Work out the finished part from the listing and answer in its coordinate system (mm). A direction names the side the tool comes from. Round coordinates to 2 decimals unless told otherwise and drop trailing zeros. Loops run counter-clockwise (first coordinate to the right, second up) from the corner with the lowest first, then second, coordinate; pieces in that order, holes last.
Autodesk Inventor part; units mm, degrees
ref_plane "YZ Plane" through (0, 0, 0) normal (1, 0, 0) x (0, 1, 0)
ref_plane "XZ Plane" through (0, 0, 0) normal (0, 1, 0) x (-1, 0, 0)
sketch "Sketch1" plane through (0, 0, 0) normal (0, 1, 0) x (-1, 0, 0)
  line L0 (-20, 10) -> (20, 10)
  line L1 (20, 10) -> (20, -10)
  line L2 (20, -10) -> (-20, -10)
  line L3 (-20, -10) -> (-20, 10)
  line L4 (-20, 10) -> (20, -10) construction
  line L5 (20, 10) -> (-20, -10) construction
  point P0 (0, 0)
  dimension "d0" = 40
  dimension "d1" = 20
extrude "Extrusion1" add sketch "Sketch1" along normal blind 37
sketch "Sketch2" plane through (0, 37, 0) normal (0, 1, 0) x (1, 0, 0)
  line L0 (20, 10) -> (-20, 10)
  line L1 (-20, 10) -> (-20, -10)
  line L2 (-20, -10) -> (20, -10)
  line L3 (20, -10) -> (20, 10)
  circle A0 centre (-10, 0) radius 10
  line L4 (-20, 10) -> (-20, -10)
  line L5 (15, -10) -> (15, 10)
  line L6 (15, 9.25) -> (-6.2003, 9.25)
  line L7 (-6.2003, -9.25) -> (15, -9.25)
  point P0 (0, 0)
  dimension "d4" = 5
extrude "Extrusion2" add sketch "Sketch2" along normal blind 2 contours A0 | L5 L7 A0 L6
sketch "Sketch3" plane through (0, 39, 0) normal (0, 1, 0) x (1, 0, 0)
  line L0 (-6.2003, -9.25) -> (15, -9.25)
  line L1 (15, -9.25) -> (15, 9.25)
  line L2 (15, 9.25) -> (-6.2003, 9.25)
  arc A0 (-6.2003, 9.25) -> (-6.2003, -9.25) centre (-10, 0) ccw
  circle A1 centre (-10, 0) radius 6.5
  point P0 (0, 0)
  dimension "d8" = 13
extrude "Extrusion3" add sketch "Sketch3" along normal blind 2 contours A1
sketch "Sketch4" plane through (-10, 41, 0) normal (0, 1, 0) x (1, 0, 0)
  circle A0 centre (0, 0) radius 6.5
  circle A1 centre (0, 0) radius 2.9
  circle A2 centre (0, 0) radius 1.5
  point P0 (10, 0)
  dimension "d11" = 5.8
  dimension "d12" = 3
extrude "Extrusion4" add sketch "Sketch4" along normal blind 4 contours A1
ref_plane "Work Plane1" through (0, 28, 0) normal (0, -1, 0) x (1, 0, 0)
sketch "Sketch5" plane through (0, 28, 0) normal (0, -1, 0) x (1, 0, 0)
  arc A0 (-10, -10) -> (-6.2003, -9.25) centre (-10, 0) ccw
  line L0 (-6.2003, -9.25) -> (15, -9.25)
  line L1 (15, -9.25) -> (15, 9.25)
  line L2 (15, 9.25) -> (-6.2003, 9.25)
  arc A1 (-6.2003, 9.25) -> (-10, 10) centre (-10, 0) ccw
  line L3 (-10, 10) -> (20, 10)
  line L4 (20, 10) -> (20, -10)
  line L5 (20, -10) -> (-10, -10)
  arc A2 (-10, 10) -> (-20, 0) centre (-10, 0) ccw
  line L6 (-20, 0) -> (-20, 10)
  line L7 (-20, 10) -> (-10, 10)
  arc A3 (-20, 0) -> (-10, -10) centre (-10, 0) ccw
  line L8 (-10, -10) -> (-20, -10)
  line L9 (-20, -10) -> (-20, 0)
  line L10 (-20, 10) -> (-26.3, 10)
  line L11 (-26.3, 10) -> (-26.3, -10)
  line L12 (-26.3, -10) -> (-20, -10)
  line L13 (-20, -10) -> (-20, 10)
  line L14 (20, 10) -> (26.3, 10)
  line L15 (26.3, 10) -> (26.3, -10)
  line L16 (26.3, -10) -> (20, -10)
  line L17 (20, -10) -> (20, 10)
  circle A4 centre (24.3, 5.8) radius 2.2
  line L18 (20, 5.8) -> (22.1, 5.8) construction
  line L19 (0, -10) -> (0, -15.1491)
  line L20 (20, 10) -> (20, -10)
  line L21 (20, 0) -> (22.5191, 0)
  line L22 (24.3, 8) -> (24.3, 10) construction
  circle A5 centre (24.3, -5.8) radius 2.2
  circle A6 centre (-24.3, 5.8) radius 2.2
  circle A7 centre (-24.3, -5.8) radius 2.2
  point P0 (0, 0)
  point P1 (26.3, -6.7165)
  point P2 (26.3, -4.8835)
  point P3 (26.3, 4.8835)
  point P4 (26.3, 6.7165)
  point P5 (-26.3, 6.7165)
  point P6 (-26.3, 4.8835)
  point P7 (-26.3, -4.8835)
  point P8 (-26.3, -6.7165)
  point P9 (-20, 0)
  dimension "d16" = 6.3
  dimension "d17" = 6.3
  dimension "d18" = 4.4
  dimension "d19" = 2.1
  dimension "d20" = 2
extrude "Extrusion5" add sketch "Sketch5" against normal blind 2.45 contours L9 L12 L11 A7 A6 L10 L6 | L4 L14 L15 A4 A5 L16
equation "\"d16\" = d17"
properties part number "MG996R"
1. Consider probe 1 along Z at (x, y) = (24.3, 28.6); probe 2 along Z at (x, y) = (-10, 44); probe 3 along Y at (x, z) = (4.5, -7.75). Determine where each line is inside the solid, lowest interval first.
Answer key:
probe 1: z = -10 to -8, -3.6 to 3.6, 8 to 10
probe 2: z = -2.9 to -1.5, 1.5 to 2.9
probe 3: y = 0 to 39
2. Determine the mould class of faces 6 (the face through (-20, 34, 0)), 7 (the face through (-22.1, 29.21, 5.72)), 8 (the face through (22, 28, 0)) for opening direction X: +X half, -X half, draft (parallel to the pull), parting line (faces both ways), or undercut.
Answer key:
face 6: -X half
face 7: undercut
face 8: draft
3. Given pin 1 (8 mm diameter, centred on x = -17.5, z = 7, fed in from +Y); pin 2 (6 mm diameter, centred on y = 18.5, z = 3, fed in from +X); pin 3 (6 mm diameter, centred on x = 9, z = -7.5, fed in from +Y); pin 4 (2.5 mm diameter, centred on x = 24.3, z = -5.8, fed in from +Y), each flat-ended and moving along its own axis, determine where each tip first touches the part or whether it passes through.
Answer key:
pin 1: stops at y = 41
pin 2: stops at x = 20
pin 3: stops at y = 39
pin 4: passes through
4. Which of the six approach directions +Z, -Z, +X, -X, +Y, -Y give full straight-line access (tool end or side, diameter ignored) to faces 1 (the face through (22, 30.45, 0)), 2 (the face through (-22, 30.45, 0)), 3 (the face through (4, 38, 9.25)), 4 (the face through (-12.9, 43, 0.1)), 5 (the face through (-18, 37, -8))?
Answer key:
face 1: +Z, -Z, +X, +Y
face 2: +Z, -Z, -X, +Y
face 3: +Z, +X, +Y
face 4: +Y
face 5: -Z, -X, +Y
5. Find section A-A (x = -24.3). Write down the section's boundary in (y, z).
Answer key:
outline: (28, -10) - (30.45, -10) - (30.45, -8) - (28, -8) - close; (28, -3.6) - (30.45, -3.6) - (30.45, 3.6) - (28, 3.6) - close; (28, 8) - (30.45, 8) - (30.45, 10) - (28, 10) - close
6. Find section C-C (y = 24). Write down the section's boundary in (x, z), then the cut area to 3 significant figures.
Answer key:
outline: (-20, -10) - (20, -10) - (20, 10) - (-20, 10) - close
area: 800 mm2
7. Find section B-B (x = 6). Write down the section's boundary in (y, z), then the cut area to 3 significant figures.
Answer key:
outline: (0, -10) - (37, -10) - (37, -9.25) - (39, -9.25) - (39, 9.25) - (37, 9.25) - (37, 10) - (0, 10) - close
area: 777 mm2
8. Find section D-D (z = -5.8). Write down the section's boundary in (x, y).
Answer key:
outline: (-22.1, 28) - (-20, 28) - (-20, 0) - (20, 0) - (20, 28) - (22.1, 28) - (22.1, 30.45) - (20, 30.45) - (20, 37) - (15, 37) - (15, 39) - (-7.07, 39) - (-7.07, 41) - (-12.93, 41) - (-12.93, 39) - (-18.15, 39) - (-18.15, 37) - (-20, 37) - (-20, 30.45) - (-22.1, 30.45) - close
